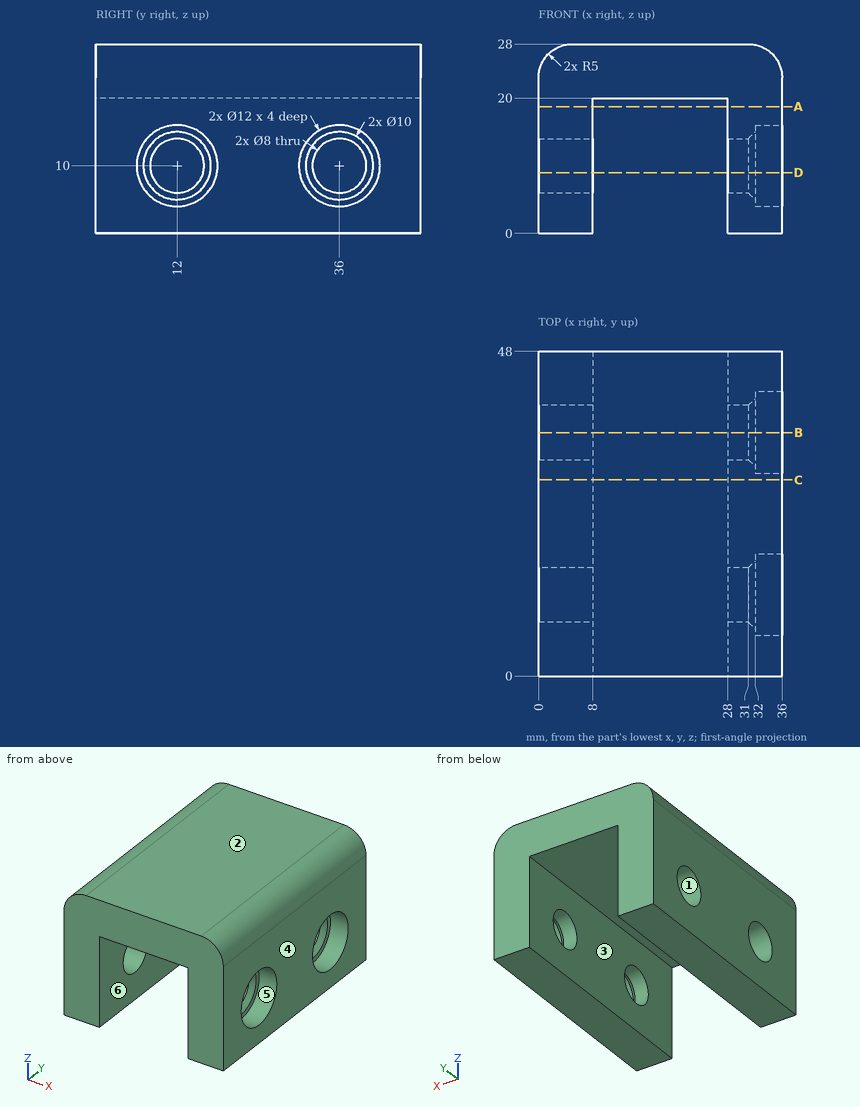
Could you check a few things on this drawing? It's one solid part, dimensions in mm from its lowest x, y, z. A direction names the side the tool comes from. Coordinates: 2 decimals unless noted, no trailing zeros. Order: outer loops, then holes, each group sorted by start corner. A loop starts at its lowest first (then second) coordinate and runs counter-clockwise, first axis right, second up. Notation, with made-up numbers: (-10.5, -23) - (-2.5, -23) arc R18 ccw to (-2.5, -19) - close; hole circle Ø7 at (49, 65.25). An arc over 180 degrees is marked (long way). Answer as a JSON object with one key per item and string values. Group by question number.
Q1. Imagine slicing it at D-D (z = 9). Give the number of separate pieces and of enclosed holes in the cut face, and give its area (3 significant figures).
Q2. Will these pins go through, and if not, where does the flat tip stop? P1, Ø6, axis at y = 13.5, z = 12, coming from the +X side; P2, Ø1.5, axis at y = 33.5, z = 13, coming from the -X side; P3, Ø6, axis at x = 17, y = 22, coming from the -Z side.
Q3. Imagine slicing it at C-C (y = 29). Please give me the cut outline in (x, z), and give its area (3 significant figures).
Q4. I need wall thicknesses on line 1 (X direction, y = 17.5, z = 19); line 2 (X direction, y = 9, z = 5.75); line 3 (Z direction, x = 11.5, y = 5). Which ranges of each line are inside material? Lowest first, please. Write a range as from..to.
Q5. Imagine slicing it at A-A (z = 18.75). Please give me the cut outline in (x, y).
Q6. Imagine slicing it at B-B (y = 36). Please give me the cut outline in (x, z).
Q7. On a 3-axis mill with a long thin cutter (end or side, diameter ignored), from which of +Z, -Z, +X, -X, +Y, -Y can I reach the whole of each face in a straight line? I mean the marked faces 4, 5 and 6. Say none if no direction works.
Q8. We'd pull the mould along Z, two halves only. Please class the marked faces 1, 2 and 3: +Z half, -Z half, draft (parallel to the pull), parting line (faces both ways), or undercut.
Determined:
{
 "1": {"separate pieces": "6", "enclosed holes": "0", "area": "485 mm2"},
 "2": {"P1": "stops at x = 32", "P2": "stops at x = 0", "P3": "stops at z = 20"},
 "3": {"outline": "(0, 0) - (8, 0) - (8, 20) - (28, 20) - (28, 0) - (36, 0) - (36, 23) arc R5 ccw to (31, 28) - (5, 28) arc R5 ccw to (0, 23) - close", "area": "597 mm2"},
 "4": {"line 1": "x = 0..8, 28..36", "line 2": "x = 0..8, 28..32", "line 3": "z = 20..28"},
 "5": {"outline": "(0, 0) - (8, 0) - (8, 48) - (0, 48) - close; (28, 0) - (36, 0) - (36, 48) - (28, 48) - close"},
 "6": {"outline": "(0, 0) - (8, 0) - (8, 6) - (0, 6) - close; (0, 14) - (8, 14) - (8, 20) - (28, 20) - (28, 14) - (31, 14) - (32, 15) - (32, 16) - (36, 16) - (36, 23) arc R5 ccw to (31, 28) - (5, 28) arc R5 ccw to (0, 23) - close; (28, 0) - (36, 0) - (36, 4) - (32, 4) - (32, 5) - (31, 6) - (28, 6) - close"},
 "7": {"face 4": "+Z, -Z, +X, +Y, -Y", "face 5": "+X", "face 6": "-Z, +Y, -Y"},
 "8": {"face 1": "undercut", "face 2": "+Z half", "face 3": "draft"}
}
